Here's how the part is built. I have some questions about the finished solid (model axes, mm). A direction names the side the tool comes from. Coordinates: 2 decimals unless noted, no trailing zeros. Order: outer loops, then holes, each group sorted by start corner. A loop starts at its lowest first (then second) coordinate and runs counter-clockwise, first axis right, second up. Notation, with made-up numbers: (44, 49) - (74, 49) arc R22 ccw to (74, 58) - close; hole circle Ø6 at (24.25, 19). An arc over 180 degrees is marked (long way). Answer as CSV lines item,"result". Start each with the question number.
Q1. Suppose I cut it at B-B (x = 0). Please give me the cut outline in (y, z), then the cut area to 3 significant figures.
Q2. I need wall thicknesses on line 1 (Y direction, x = 0, z = 1.55); line 2 (Z direction, x = 4.75, y = -12.25); line 3 (X direction, y = -4.5, z = 16.5). Which ranges of each line are inside material? Lowest first, please.
Q3. For pin 1 Ø10 at (x, z) = (-8, 21.5) entering from -Y; pin 2 Ø3 at (x, y) = (-8.5, 4) entering from -Z; pin 3 Ø1.5 at (y, z) = (0.5, 19) entering from +X, each with a flat end and sliding along its axis, tell me the tip position at first contact or that it passes through.
Q4. Suppose I cut it at C-C (x = 10.5). Please give me the cut outline in (y, z).
Q5. Suppose I cut it at D-D (y = 11). Please give me the cut outline in (x, z).
Q6. Thinking about a two-plate mould opening in X: for faces 3 (the face through (-4, 7, 2)), 4 (the face through (5.29, -7.95, 1.01)), 5 (the face through (-14.985, 0.66, 0.986)), which applies, released by +X, released by -X, zero draft, split by the parting line, or undercut?
Q7. For faces 1 (the face through (-1.08, -4.88, 12.66)), 2 (the face through (-7.493, 0.33, 12.353)), which set-ups out of +Z, -Z, +X, -X, +Y, -Y let a thin tool reach every point of the face, with its end or its side?
Q8. Suppose I cut it at A-A (y = 0). Please give me the cut outline in (x, z), then the cut area to 3 significant figures.
from build123d import *

# Parameters (mm, degrees)
SKETCH1_R           = 15
BOSS_EXTRUDE1_DEPTH = 2
SKETCH2_R           = 7.5
BOSS_EXTRUDE2_DEPTH = 22
SKETCH3_R           = 5
CUT_EXTRUDE1_DEPTH  = 25
SKETCH4_R           = 2
CUT_EXTRUDE2_DEPTH  = 3
CHAMFER1_SIZE       = 1
CHAMFER2_SIZE       = 1


with BuildPart() as part:
    # Sketch1 → Boss-Extrude1 (new body)
    with BuildSketch(Plane.XY):
        Circle(SKETCH1_R)
    extrude(amount=BOSS_EXTRUDE1_DEPTH)

    # Sketch2 → Boss-Extrude2 (add)
    with BuildSketch(Plane.XY.offset(2)):
        Circle(SKETCH2_R)
    extrude(amount=BOSS_EXTRUDE2_DEPTH)

    # Sketch3 → Cut-Extrude1 (cut, through all)
    with BuildSketch(Plane.XY.offset(24)):
        Circle(SKETCH3_R)
    extrude(amount=-CUT_EXTRUDE1_DEPTH, mode=Mode.SUBTRACT)

    # Sketch4 → Cut-Extrude2 (cut, through all)
    with BuildSketch(Plane.XY.offset(2)):
        with Locations((0, 11.5)):
            Circle(SKETCH4_R)
        with Locations((10.937149937, 3.553695435)):
            Circle(SKETCH4_R)
        with Locations((6.759530401, -9.303695435)):
            Circle(SKETCH4_R)
        with Locations((-6.759530401, -9.303695435)):
            Circle(SKETCH4_R)
        with Locations((-10.937149937, 3.553695435)):
            Circle(SKETCH4_R)
    extrude(amount=-CUT_EXTRUDE2_DEPTH, mode=Mode.SUBTRACT)

    # Chamfer1
    chamfer1_edges = [part.edges().sort_by_distance(p)[0] for p in [
        (-5, 0, 0),
    ]]
    chamfer(chamfer1_edges, length=CHAMFER1_SIZE)

    # Chamfer2
    chamfer2_edges = [part.edges().sort_by_distance(p)[0] for p in [
        (-7.5, 0, 24),
    ]]
    chamfer(chamfer2_edges, length=CHAMFER2_SIZE)


solid = part.part
Here are the results:
1,outline,"(-15, 0) - (-6, 0) - (-5, 1) - (-5, 24) - (-6.5, 24) - (-7.5, 23) - (-7.5, 2) - (-15, 2) - close; (5, 1) - (6, 0) - (9.5, 0) - (9.5, 2) - (7.5, 2) - (7.5, 23) - (6.5, 24) - (5, 24) - close; (13.5, 0) - (15, 0) - (15, 2) - (13.5, 2) - close"
1,area,"140 mm²"
2,line 1,"y = -15 to -5, 5 to 9.5, 13.5 to 15"
2,line 2,"z = 0 to 2"
2,line 3,"x = -6 to -2.18, 2.18 to 6"
3,pin 1,"stops at y = -6.87"
3,pin 2,"stops at z = 0"
3,pin 3,"stops at x = 7.5"
4,outline,"(-10.71, 0) - (1.6, 0) - (1.6, 2) - (-10.71, 2) - close; (5.51, 0) - (10.71, 0) - (10.71, 2) - (5.51, 2) - close"
5,outline,"(-10.2, 0) - (-1.94, 0) - (-1.94, 2) - (-10.2, 2) - close; (1.94, 0) - (10.2, 0) - (10.2, 2) - (1.94, 2) - close"
6,face 3,"zero draft"
6,face 4,"undercut"
6,face 5,"split by the parting line"
7,face 1,"+Z, -Z"
7,face 2,"+Z"
8,outline,"(-15, 0) - (-6, 0) - (-5, 1) - (-5, 24) - (-6.5, 24) - (-7.5, 23) - (-7.5, 2) - (-15, 2) - close; (5, 1) - (6, 0) - (15, 0) - (15, 2) - (7.5, 2) - (7.5, 23) - (6.5, 24) - (5, 24) - close"
8,area,"148 mm²"
